Build history of the part. All positions in model axes, mm. Coordinates: 2 decimals unless noted, no trailing zeros. Loops run counter-clockwise (first coordinate to the right, second up) from the corner with the lowest first, then second, coordinate; pieces in that order, holes last.
(1) Wall check: L1, parallel to X at y = 33, z = 21; L2, parallel to X at y = 3, z = 21.5; L3, parallel to Y at x = 13, z = 2. Give the ranges that are in metal, low to high.
(2) Slice it at B-B (y = -21.5). Give the cut face in (x, z).
(3) Slice it at A-A (z = 19.5). Give the cut face in (x, y).
(4) Flat gauge pins, fed straight in: P1, Ø1.5, axis at y = 17.5, z = 26, coming from the -X side; P2, Ø12, axis at y = 30, z = 29.5, coming from the +X side; P3, Ø1.5, axis at y = 33, z = 39.5, coming from the -X side. Where does each tip first touch, or does it go through?
from build123d import *

# Parameters (mm, degrees)
EXTRUSION1_DEPTH      = 60
EXTRUSION1_DEPTH_BACK = 1


with BuildPart() as part:
    # Esquisse1 → Extrusion1 (new, two sides: drawn at the far end of the back side and taken through both)
    with BuildSketch(Plane.XY.offset(-EXTRUSION1_DEPTH_BACK)):
        with BuildLine():
            Line((-356.481440216, -16.365912372), (-335.479161402, -39.691306064))
            ThreePointArc((-335.479161402, -39.691306064), (-332.115079578, -42.135454576), (-328.047713147, -43))
            Line((-328.047713147, -43), (0, -43))
            ThreePointArc((0, -43), (43, 0), (0, 43))
            Line((0, 43), (-317.5, 43))
            ThreePointArc((-317.5, 43), (-352.076517488, 25.562950503), (-358.610595586, -12.60630519))
            ThreePointArc((-358.610595586, -12.60630519), (-357.751492884, -14.602474173), (-356.481440216, -16.365912372))
        make_face()
    extrude(amount=EXTRUSION1_DEPTH + EXTRUSION1_DEPTH_BACK)


solid = part.part
Response values:
1. L1: x = -345.07 to 27.57
1. L2: x = -360.4 to 42.9
1. L3: y = -40.99 to 40.99
2. outline: (-351.86, -1) - (37.24, -1) - (37.24, 60) - (-351.86, 60) - close
3. outline: (-358.61, -12.61) arc R10 ccw to (-356.48, -16.37) - (-335.48, -39.69) arc R10 ccw to (-328.05, -43) - (0, -43) arc R43 ccw to (0, 43) - (-317.5, 43) arc R43 ccw to start
4. P1: stops at x = -357.1
4. P2: stops at x = 35.68
4. P3: stops at x = -345.94
